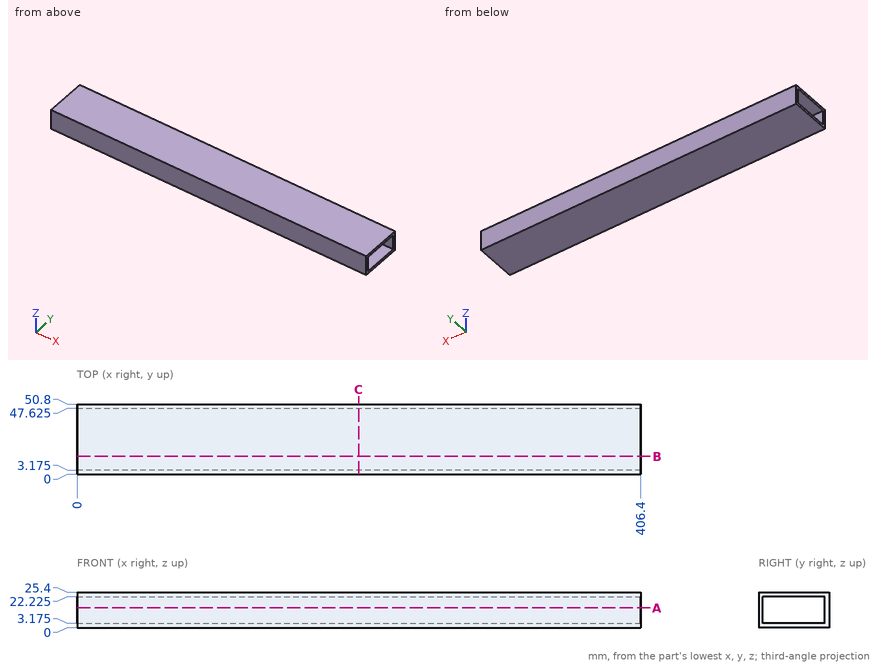
Design review of the part shown in the three views and the two pictorial views. Dimensions are in mm from the part's minimum x, y and z. Round coordinates to 2 decimals unless told otherwise and drop trailing zeros. Write each loop counter-clockwise with the first axis right and the second up, starting at its lowest first coordinate (ties: lowest second). Pieces come first, ordered by that corner, then holes. Notation, with made-up numbers: (-19, 33) -> (-14, 33) arc R16 cw to (-14, 54) -> close; hole circle Ø1 at (69, 31). An arc over 180 degrees is marked (long way). One line per question, with ' | ' between items. Start each with the question number.
1) Add section A-A (z = 14.25). Write out the cut boundary in (x, y) (3 decimals).
2) Add section C-C (x = 203). Write out the cut boundary in (y, z) (3 decimals).
3) Add section B-B (y = 13). Write out the cut boundary in (x, z) (3 decimals).
4) Wall thickness on line 1 along Z through (x, y) = (129, 15) (3 decimals); line 2 along Y through (x, z) = (182, 22) (3 decimals): over which ranges is each line inside the solid? List them lowest first.
Reported:
1) outline: (0, 0) -> (406.4, 0) -> (406.4, 3.175) -> (0, 3.175) -> close; (0, 47.625) -> (406.4, 47.625) -> (406.4, 50.8) -> (0, 50.8) -> close
2) outline: (0, 0) -> (50.8, 0) -> (50.8, 25.4) -> (0, 25.4) -> close; hole (3.175, 3.175) -> (47.625, 3.175) -> (47.625, 22.225) -> (3.175, 22.225) -> close
3) outline: (0, 0) -> (406.4, 0) -> (406.4, 3.175) -> (0, 3.175) -> close; (0, 22.225) -> (406.4, 22.225) -> (406.4, 25.4) -> (0, 25.4) -> close
4) line 1: z = 0 to 3.175, 22.225 to 25.4 | line 2: y = 0 to 3.175, 47.625 to 50.8
